Design review of the part built by this model. Coordinates are the model's own, in mm. Face numbers are marked on the shaded views. A direction names the side the tool comes from. Round coordinates to 2 decimals unless told otherwise and drop trailing zeros. Write each loop counter-clockwise with the first axis right and the second up, starting at its lowest first coordinate (ties: lowest second). Pieces come first, ordered by that corner, then holes. Notation, with made-up numbers: M -36.75,83.5 L 11.25,83.5 A14 ccw 11.25,90.5 Z; hole C 26.5,-22.5 d9. An arc over 180 degrees is marked long. One line per question, with ' | ' between items. Start each with the question number.
Item 1: Add section A-A, the plane z = 0. State the section outline as (x, y) points, and give its area (3 significant figures).
Item 2: For L1, parallel to X at y = 64.5, z = -0.5; L2, parallel to Y at x = 7.5, z = -11.5; L3, parallel to Y at x = -7.5, z = 3, list the stretches that pass through material, from the lowest coordinate up.
Item 3: Machinability: for the marked faces 1 and 2, which of the approach directions +Z, -Z, +X, -X, +Y, -Y give a long, thin tool a straight path to every point of the face, cutting with its end or side? Answer none if there is none.
Item 4: Insertion check: pin 1 Ø1.5 at (y, z) = (30.5, -4) entering from +X; pin 2 Ø1.5 at (y, z) = (66, 10.5) entering from -X; pin 3 Ø4 at (y, z) = (71.5, 13.5) entering from +X; pin 4 Ø2 at (y, z) = (134, -1) entering from +X. Each pin has a flat end and moves straight along its axis. Give the tip position at first contact, or say it passes through.
Item 5: Add section B-B, the plane x = 0. State the section outline as (y, z) points.
Item 6: Add section C-C, the plane y = 132. State the section outline as (x, z) points.
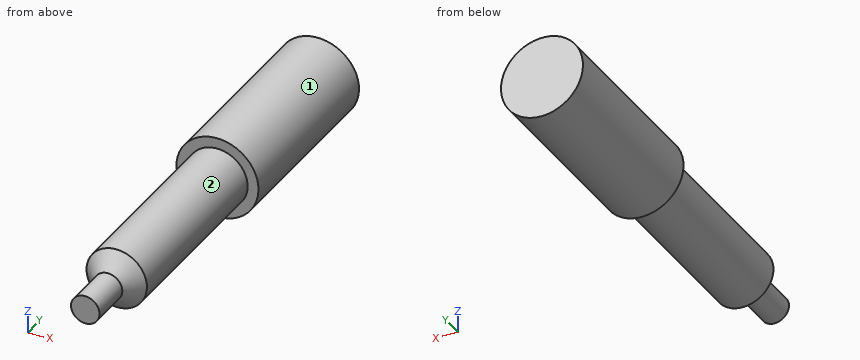
```python
from build123d import *

# Parameters (mm, degrees)
SKETCH2_W     = 12.720955
SKETCH2_H     = 33.02
SKETCH2_W_2   = 5.999999938
SKETCH2_H_2   = 25.4
CHAMFER1_SIZE = 7.62


with BuildPart() as part:
    # Sketch2 → Revolve1 (revolve)
    with BuildSketch(Plane.XY, mode=Mode.PRIVATE) as revolve1_sk:
        with Locations((6.3604775, 86.36)):
            Rectangle(SKETCH2_W, SKETCH2_H)
        Polygon((0, 181.102), (0, 102.87), (12.720955, 102.87), (17.272, 102.87), (17.272, 181.102), align=None)
        Polygon((0, 69.85), (0, 25.4), (5.999999938, 25.4), (12.720955, 25.4), (12.720955, 69.85), align=None)
        with Locations((2.999999969, 12.7)):
            Rectangle(SKETCH2_W_2, SKETCH2_H_2)
    revolve(revolve1_sk.sketch.rotate(Axis((0, 0, 0), (0, 1, 0)), 90), axis=Axis((0, 0, 0), (0, 1, 0)))

    # Chamfer1
    # the kernel refuses this chamfer: 7.62 mm, written as the material it adds along each edge
    with BuildSketch(Plane(origin=(0, 25.4, 0), x_dir=(0, 0, -1), z_dir=(1, 0, 0))) as chamfer1_piece_1_section:
        Polygon((5.999999938 + CHAMFER1_SIZE, 0), (5.999999938, -CHAMFER1_SIZE), (5.999999938, 0), align=None)
    chamfer1_piece_1 = revolve(axis=Axis((0, 25.4, 0), (0, 1, 0)), mode=Mode.PRIVATE)
    chamfer1_piece_1 = chamfer1_piece_1 & Plane(origin=(0, 21.11622986, 0), x_dir=(0, 0, -1), z_dir=(0, 1, 0)) * Cylinder(12.720955, 55, mode=Mode.PRIVATE)
    add(chamfer1_piece_1)


solid = part.part
```
Computed values:
1) outline: M -17.27,102.87 L -12.72,102.87 L -12.72,24.5 L -6,17.78 L -6,0 L 6,0 L 6,17.78 L 12.72,24.5 L 12.72,102.87 L 17.27,102.87 L 17.27,181.1 L -17.27,181.1 Z | area: 5,040 mm^2
2) L1: x = -12.71 to 12.71 | L2: y = 102.87 to 181.1 | L3: y = 19.86 to 181.1
3) face 1: +Y, -Y | face 2: -Y
4) pin 1: stops at x = 12.3 | pin 2: stops at x = -8.17 | pin 3: stops at x = 5.44 | pin 4: stops at x = 17.27
5) outline: M 0,-6 L 17.78,-6 L 24.5,-12.72 L 102.87,-12.72 L 102.87,-17.27 L 181.1,-17.27 L 181.1,17.27 L 102.87,17.27 L 102.87,12.72 L 24.5,12.72 L 17.78,6 L 0,6 Z
6) outline: C 0,0 d34.54
